Source: CAD feature listing. Evaluate the final solid. Frame: model axes, mm. Face numbers are marked on the shaded views. A direction names the side the tool comes from. Coordinates: 2 decimals unless noted, no trailing zeros. Loops run counter-clockwise (first coordinate to the right, second up) from the corner with the lowest first, then second, coordinate; pieces in that order, holes last.
from build123d import *

# Parameters (mm, degrees)
F1_DEPTH = 15
F3_D     = 6


with BuildPart() as f1:
    # F0 (on Top) → F1 (new body)
    with BuildSketch(Plane.XY):
        Polygon((67.5, -12.5), (67.5, 12.5), (-67.5, 12.5), (-67.5, -12.5), (-34.5, -12.5), (-34.5, -4.5), (-24.5, -4.5), (-24.5, -12.5), (-18.5, -12.5), (-18.5, 7.5), (21.5, 7.5), (21.5, -8.5), (1.5, -8.5), (1.5, -12.5), (41.5, -12.5), (41.5, -4.5), (51.5, -4.5), (51.5, -12.5), align=None)
    extrude(amount=F1_DEPTH)

    # F3 (through all)
    with Locations(Plane.XY.offset(15)):
        with Locations((-52.5, 2.5), (-40.5, 2.5), (59.5, 2.5)):
            Hole(F3_D / 2)


solid = f1.part
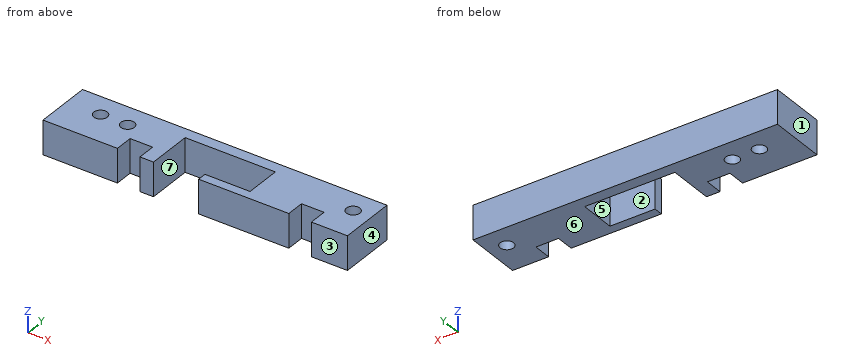
Q1. Section C-C, the plane y = 2.5. Return the cut outline in (x, z), plus the area to 4 significant figures.
Q2. Draft query along X for the marked faces 1, 2, 3 and 4. Return one class per face: +X half, -X half, draft (parallel to the pull), parting line (faces both ways), or undercut.
Q3. Section A-A, the plane z = 13.5. Return the cut outline in (x, y).
Q4. Section D-D, the plane x = 4. Return the cut outline in (y, z).
Q5. Contact query for flat-ended pins moving along their axis: pin 1 Ø8 at (x, z) = (-12, 3.5) entering from -Y; pin 2 Ø3 at (x, z) = (-30.5, 5) entering from -Y. Output: stop coordinate, or through.
Q6. Line query: line 1 along X through (y, z) = (3.5, 2.25); line 2 along Y through (x, z) = (-52.5, 3.5); line 3 along X through (y, z) = (-1.25, 9.25). Output: solid intervals per line, ascending.
Q7. Section B-B, the plane x = -52.5. Return the cut outline in (y, z).
Q8. Access query for the marked faces 5, 6 and 7. Directions: +Z, -Z, +X, -X, +Y, -Y. A direction counts if a zero-diameter tool reaches every point of the face in a straight line with its end or side. Return the directions, or none.
Derived:
1. outline: (-67.5, 0) - (-55.5, 0) - (-55.5, 15) - (-67.5, 15) - close; (-49.5, 0) - (-43.5, 0) - (-43.5, 15) - (-49.5, 15) - close; (-37.5, 0) - (-18.5, 0) - (-18.5, 15) - (-37.5, 15) - close; (21.5, 0) - (56.5, 0) - (56.5, 15) - (21.5, 15) - close; (62.5, 0) - (67.5, 0) - (67.5, 15) - (62.5, 15) - close
1. area: 1,155 mm2
2. face 1: -X half
2. face 2: undercut
2. face 3: draft
2. face 4: +X half
3. outline: (-67.5, -12.5) - (-34.5, -12.5) - (-34.5, -4.5) - (-24.5, -4.5) - (-24.5, -12.5) - (-18.5, -12.5) - (-18.5, 7.5) - (21.5, 7.5) - (21.5, -8.5) - (1.5, -8.5) - (1.5, -12.5) - (41.5, -12.5) - (41.5, -4.5) - (51.5, -4.5) - (51.5, -12.5) - (67.5, -12.5) - (67.5, 12.5) - (-67.5, 12.5) - close; hole circle Ø6 at (-52.5, 2.5); hole circle Ø6 at (-40.5, 2.5); hole circle Ø6 at (59.5, 2.5)
4. outline: (-12.5, 0) - (-8.5, 0) - (-8.5, 15) - (-12.5, 15) - close; (7.5, 0) - (12.5, 0) - (12.5, 15) - (7.5, 15) - close
5. pin 1: stops at y = 7.5
5. pin 2: stops at y = -4.5
6. line 1: x = -67.5 to -55.33, -49.67 to -43.33, -37.67 to -18.5, 21.5 to 56.67, 62.33 to 67.5
6. line 2: y = -12.5 to -0.5, 5.5 to 12.5
6. line 3: x = -67.5 to -18.5, 21.5 to 67.5
7. outline: (-12.5, 0) - (-0.5, 0) - (-0.5, 15) - (-12.5, 15) - close; (5.5, 0) - (12.5, 0) - (12.5, 15) - (5.5, 15) - close
8. face 5: +Z, -Z
8. face 6: -Z, +X, -X, +Y, -Y
8. face 7: +Z, -Z, -Y
